For this review, take the finished solid that the model builds, in its own axes (mm). A direction names the side the tool comes from. Round coordinates to 2 decimals unless told otherwise and drop trailing zeros. Loops run counter-clockwise (first coordinate to the right, second up) from the corner with the lowest first, then second, coordinate; pieces in that order, holes last. Notation, with made-up numbers: (-26, 79) -> (11, 79) arc R20 cw to (11, 92) -> close; hole circle Ø8 at (-8, 8.25). An arc over 180 degrees is marked (long way). One line per question, with ' | ' between items. Start each with the question number.
1. For pin 1 Ø12 at (y, z) = (8, 7) entering from +X; pin 2 Ø3 at (y, z) = (12.85, 11.91) entering from -X; pin 3 Ø6 at (x, z) = (13, 13.5) entering from +Y; pin 4 Ø1 at (x, z) = (-1, 12) entering from -Y, all flat-tipped, find the tip position at first contact; note any pin that passes through.
2. Wall thickness on line 1 along X through (y, z) = (13, 21.25) (3 decimals); line 2 along Y through (x, z) = (9.25, 13.75); line 3 along Y through (x, z) = (-1.5, 9.75): over which ranges is each line inside the solid? List them lowest first.
3. Consider section D-D (z = 2). Write out the cut boundary in (x, y) (1 decimal), and give its area (3 significant figures).
4. Consider section A-A (x = 8.5). Write out the cut boundary in (y, z), and give its area (3 significant figures).
5. For faces 1 (the face through (13, -15.157, 12)), 2 (the face through (12.7, -16.7, 7.2)), list the 3-axis set-ups (+Z, -Z, +X, -X, +Y, -Y) from which the entire face can be reached by the end or side of a thin tool; tool diameter is ignored.
6. Consider section C-C (z = 11.5). Write out the cut boundary in (x, y) (1 decimal).
7. Draft analysis for pull direction Z (two halves, no side actions). For faces 3 (the face through (-1.61, 11.753, 9.794)), 4 (the face through (-1.57, 19.27, 23.05)), 5 (the face through (0, 7, 12)), 6 (the face through (16.699, -16.766, 0.724)), state which applies: pulls with the +Z half, pulls with the -Z half, needs draft (parallel to the pull), parting line crosses it, or undercut.
8. Consider section B-B (y = 14.5). Write out the cut boundary in (x, z) (1 decimal).
```python
from build123d import *

# Parameters (mm, degrees)
BOSS_EXTRUDE1_DEPTH = 23.8125
SKETCH5_R           = 2.38125
CUT_EXTRUDE2_DEPTH  = 3.175
CUT_EXTRUDE3_REACH  = 47.909
SKETCH8_R           = 2.38125
FILLET1_R           = 2.54


with BuildPart() as part:
    # Sketch1 → Boss-Extrude1 (new body)
    with BuildSketch(Plane.XY):
        with BuildLine():
            Line((0, 19.99549417), (0, -7.21908183))
            ThreePointArc((0, -7.21908183), (2.324839924, -12.831741905), (7.9375, -15.15658183))
            Line((7.9375, -15.15658183), (17.4625, -15.15658183))
            Line((17.4625, -15.15658183), (17.4625, -18.33158183))
            Line((17.4625, -18.33158183), (7.9375, -18.33158183))
            ThreePointArc((7.9375, -18.33158183), (0.079775894, -15.076805936), (-3.175, -7.21908183))
            Line((-3.175, -7.21908183), (-3.175, 19.99549417))
            Line((-3.175, 19.99549417), (0, 19.99549417))
        make_face()
    extrude(amount=BOSS_EXTRUDE1_DEPTH)

    # Sketch5 → Cut-Extrude2 (cut)
    with BuildSketch(Plane.ZY.offset(3.175)):
        with Locations(Location((11.90625, 12.85174417, 0), (0, 0, 270))):
            Circle(SKETCH5_R)
    extrude(amount=-CUT_EXTRUDE2_DEPTH, mode=Mode.SUBTRACT)

    # Sketch8 → Cut-Extrude3 (cut, up to next)
    with BuildSketch(Plane(origin=(0, -15.15658183, 0), x_dir=(1, 0, 0), z_dir=(0, 1, 0)), mode=Mode.PRIVATE) as cut_extrude3_sk1:
        with Locations(Location((10.31875, -7.14375, 0), (0, 0, 180))):
            Circle(SKETCH8_R)
    cut_extrude3_tool1 = extrude(cut_extrude3_sk1.sketch, amount=-CUT_EXTRUDE3_REACH, mode=Mode.PRIVATE) & part.part
    # Sketch8 → Cut-Extrude3 (cut, up to next)
    with BuildSketch(Plane(origin=(0, -15.15658183, 0), x_dir=(1, 0, 0), z_dir=(0, 1, 0)), mode=Mode.PRIVATE) as cut_extrude3_sk2:
        with Locations(Location((10.31875, -16.66875, 0), (0, 0, 180))):
            Circle(SKETCH8_R)
    cut_extrude3_tool2 = extrude(cut_extrude3_sk2.sketch, amount=-CUT_EXTRUDE3_REACH, mode=Mode.PRIVATE) & part.part
    add(cut_extrude3_tool1.solids().sort_by_distance((10.31875, -15.156582, 7.14375))[0], mode=Mode.SUBTRACT)
    add(cut_extrude3_tool2.solids().sort_by_distance((10.31875, -15.156582, 16.66875))[0], mode=Mode.SUBTRACT)

    # Fillet1
    fillet1_edges = [part.edges().sort_by_distance(p)[0] for p in [
        (-1.5875, 19.99549417, 0),
        (17.4625, -16.74408183, 23.8125),
        (-1.5875, 19.99549417, 23.8125),
        (17.4625, -16.74408183, 0),
    ]]
    fillet(fillet1_edges, radius=FILLET1_R)


solid = part.part
```
Answer block:
1) pin 1: stops at x = 0 | pin 2: passes through | pin 3: stops at y = -15.16 | pin 4: stops at y = -14.45
2) line 1: x = -3.175 to 0 | line 2: y = -18.33 to -15.16 | line 3: y = -13.09 to 11.84, 13.86 to 20
3) outline: (-3.2, -7.2) arc R11.1 ccw to (7.9, -18.3) -> (17.4, -18.3) -> (17.4, -15.2) -> (7.9, -15.2) arc R7.9 cw to (0, -7.2) -> (0, 19.9) -> (-3.2, 19.9) -> close | area: 164 mm2
4) outline: (-18.33, 0) -> (-15.16, 0) -> (-15.16, 5.61) -> (-18.33, 5.61) -> close; (-18.33, 8.68) -> (-15.16, 8.68) -> (-15.16, 15.13) -> (-18.33, 15.13) -> close; (-18.33, 18.21) -> (-15.16, 18.21) -> (-15.16, 23.81) -> (-18.33, 23.81) -> close | area: 56.1 mm2
5) face 1: +Z, -Z, +X, +Y | face 2: +Y, -Y
6) outline: (-3.2, -7.2) arc R11.1 ccw to (7.9, -18.3) -> (17.5, -18.3) -> (17.5, -15.2) -> (7.9, -15.2) arc R7.9 cw to (0, -7.2) -> (0, 10.5) -> (-3.2, 10.5) -> close; (-3.2, 15.2) -> (0, 15.2) -> (0, 20) -> (-3.2, 20) -> close
7) face 3: undercut | face 4: pulls with the +Z half | face 5: needs draft | face 6: pulls with the -Z half
8) outline: (-3.2, 0) -> (0, 0) -> (0, 10.2) -> (-3.2, 10.2) -> close; (-3.2, 13.6) -> (0, 13.6) -> (0, 23.8) -> (-3.2, 23.8) -> close
